Design review of the part built by this model. Coordinates are the model's own, in mm. A direction names the side the tool comes from. Coordinates: 2 decimals unless noted, no trailing zeros. Loops run counter-clockwise (first coordinate to the right, second up) from the corner with the lowest first, then second, coordinate; pieces in that order, holes last. Notation, with made-up numbers: (-7.5, -24) -> (41.5, -24) arc R26 cw to (41.5, 13) -> close; hole circle Ø10 at (2.5, 0.25). An arc over 180 degrees is marked (long way). Use a Markdown table: item, result. Add a question column.
Q1. Draft analysis for pull direction Z (two halves, no side actions). For faces 5 (the face through (-18.66, -201.37, -54.34)), 6 (the face through (-15.28, -209.38, -38.51)), 7 (the face through (-18.459, -209, -43)), state which applies: pulls with the +Z half, pulls with the -Z half, needs draft (parallel to the pull), parting line crosses it, or undercut.
Q2. Take a section at C-C on x = -14.5. Write out the cut boundary in (y, z).
Q3. Clearance check with flat-ended pins moving along their axes: pin 1 Ø3 at (x, z) = (-15, -40.5) entering from +Y; pin 2 Ø4 at (y, z) = (-213, -53.24) entering from +X; pin 3 Ø1.6 at (x, z) = (-17.5, -53) entering from -Y; pin 4 Ø3 at (y, z) = (-210.8, -39.24) entering from +X. State where each tip first meets the part, or that it passes through.
Q4. For faces 1 (the face through (-26.009, -211, -41)), 2 (the face through (-18.9, -210, -53.4)), 3 (the face through (-20.2, -203.8, -53.8)), 4 (the face through (-16.332, -203.496, -52.893)), list the 3-axis set-ups (+Z, -Z, +X, -X, +Y, -Y) from which the entire face can be reached by the end or side of a thin tool; tool diameter is ignored.
Q5. Take a section at D-D on z = -61.25. Write out the cut boundary in (x, y).
Q6. Take a section at A-A on y = -210.8. Write out the cut boundary in (x, z).
Q7. Take a section at B-B on z = -39. Write out the cut boundary in (x, y), plus the area to 3 significant figures.
Q8. For probe 1 along X at (y, z) = (-213.5, -39); probe 2 along Z at (x, y) = (-23.75, -210.8); probe 3 along Y at (x, z) = (-16.5, -58.25), list the stretches that pass through material, from the lowest coordinate up.
from build123d import *

# Parameters (mm, degrees)
MAIN_PROFILE_SKETCH_R          = 1.15
MAIN_EXTRUSION_DEPTH           = 3.6
DETAIL_PROFILE_2_SKETCH_R      = 2.7
DETAIL_EXTRUSION_2_DEPTH       = 0.6
DETAIL_PROFILE_3_SKETCH_R      = 1.15
DETAIL_EXTRUSION_3_DEPTH       = 2.2
DETAIL_EXTRUSION_4_DEPTH       = 1.2
DETAIL_EXTRUSION_5_DEPTH       = 2.8
DETAIL_EXTRUSION_6_DEPTH       = 4.4
ADAPTER_CROSS_BORE_1_PROFILE_R = 1.8
ADAPTER_CROSS_BORE_1_DEPTH     = 28
ADAPTER_CROSS_BORE_2_PROFILE_R = 1.6
ADAPTER_CROSS_BORE_2_DEPTH     = 16


with BuildPart() as part:
    # Main Profile Sketch → Main Extrusion (new body)
    with BuildSketch(Plane(origin=(0, -199.6, 0), x_dir=(-1, 0, 0), z_dir=(0, -1, 0))):
        with Locations(Location((19.009182883, 53.244882879, 0), (0, 0, 90))):
            Circle(MAIN_PROFILE_SKETCH_R)
    extrude(amount=MAIN_EXTRUSION_DEPTH)

    # Detail Profile 2 Sketch → Detail Extrusion 2 (add)
    with BuildSketch(Plane(origin=(0, -203.2, 0), x_dir=(-1, 0, 0), z_dir=(0, -1, 0))):
        with Locations(Location((19.009182883, 53.244882879, 0), (0, 0, 90))):
            Circle(DETAIL_PROFILE_2_SKETCH_R)
    extrude(amount=DETAIL_EXTRUSION_2_DEPTH)

    # Detail Profile 3 Sketch → Detail Extrusion 3 (add)
    with BuildSketch(Plane(origin=(0, -203.8, 0), x_dir=(-1, 0, 0), z_dir=(0, -1, 0))):
        with Locations(Location((19.009182883, 53.244882879, 0), (0, 0, 90))):
            Circle(DETAIL_PROFILE_3_SKETCH_R)
    extrude(amount=DETAIL_EXTRUSION_3_DEPTH)

    # Detail Profile 4 Sketch → Detail Extrusion 4 (add)
    with BuildSketch(Plane(origin=(0, -206, 0), x_dir=(-1, 0, 0), z_dir=(0, -1, 0))):
        with BuildLine():
            Line((18.459182883, 53.244882879), (18.459182883, 40.756988741))
            ThreePointArc((18.459182883, 40.756988741), (19.009182883, 65.744882879), (19.559182883, 40.756988741))
            Line((19.559182883, 40.756988741), (19.559182883, 53.244882879))
            Line((19.559182883, 53.244882879), (18.459182883, 53.244882879))
        make_face()
    extrude(amount=DETAIL_EXTRUSION_4_DEPTH)

    # Detail Profile 5 Sketch → Detail Extrusion 5 (add)
    with BuildSketch(Plane(origin=(0, -207.2, 0), x_dir=(-1, 0, 0), z_dir=(0, -1, 0))):
        with BuildLine():
            Line((12.009182883, 42.88872529), (12.009182883, 36.444882879))
            Line((12.009182883, 36.444882879), (18.459182883, 36.444882879))
            Line((18.459182883, 36.444882879), (18.459182883, 53.244882879))
            Line((18.459182883, 53.244882879), (19.559182883, 53.244882879))
            Line((19.559182883, 53.244882879), (19.559182883, 36.444882879))
            Line((19.559182883, 36.444882879), (26.009182883, 36.444882879))
            Line((26.009182883, 36.444882879), (26.009182883, 42.88872529))
            ThreePointArc((26.009182883, 42.88872529), (19.009182883, 65.744882879), (12.009182883, 42.88872529))
        make_face()
    extrude(amount=DETAIL_EXTRUSION_5_DEPTH)

    # Detail Profile 6 Sketch → Detail Extrusion 6 (add)
    with BuildSketch(Plane(origin=(0, -210, 0), x_dir=(-1, 0, 0), z_dir=(0, -1, 0))):
        with BuildLine():
            Line((12.009182883, 42.88872529), (12.009182883, 36.444882879))
            Line((12.009182883, 36.444882879), (18.459182883, 36.444882879))
            Line((18.459182883, 36.444882879), (18.459182883, 44.261704154))
            ThreePointArc((18.459182883, 44.261704154), (19.009182883, 62.244882879), (19.559182883, 44.261704154))
            Line((19.559182883, 44.261704154), (19.559182883, 36.444882879))
            Line((19.559182883, 36.444882879), (26.009182883, 36.444882879))
            Line((26.009182883, 36.444882879), (26.009182883, 42.88872529))
            ThreePointArc((26.009182883, 42.88872529), (19.009182883, 65.744882879), (12.009182883, 42.88872529))
        make_face()
    extrude(amount=DETAIL_EXTRUSION_6_DEPTH)

    # Adapter Cross Bore 1 profile → Adapter Cross Bore 1 (cut)
    with BuildSketch(Plane(origin=(-33.009182883, 0, 0), x_dir=(0, 0, -1), z_dir=(1, 0, 0))):
        with Locations((53.244882879, -213)):
            Circle(ADAPTER_CROSS_BORE_1_PROFILE_R)
    extrude(amount=ADAPTER_CROSS_BORE_1_DEPTH, mode=Mode.SUBTRACT)

    # Adapter Cross Bore 2 profile → Adapter Cross Bore 2 (cut)
    with BuildSketch(Plane(origin=(-27.009182883, 0, 0), x_dir=(0, 0, -1), z_dir=(1, 0, 0))):
        with Locations(Location((39.244882879, -210.8, 0), (0, 0, 180))):
            Circle(ADAPTER_CROSS_BORE_2_PROFILE_R)
    extrude(amount=ADAPTER_CROSS_BORE_2_DEPTH, mode=Mode.SUBTRACT)


solid = part.part
Answer list:
| question | item | result |
|---|---|---|
| 1 | face 5 | parting line crosses it |
| 1 | face 6 | undercut |
| 1 | face 7 | needs draft |
| 2 | outline | (-214.4, -64.9) -> (-206, -64.9) -> (-206, -41.59) -> (-207.2, -41.59) -> (-207.2, -36.44) -> (-214.4, -36.44) -> (-214.4, -45.46) -> (-210, -45.46) -> (-210, -61.03) -> (-214.4, -61.03) -> close; hole circle Ø3.2 at (-210.8, -39.24) |
| 3 | pin 1 | y = -206 |
| 3 | pin 2 | x = -6.51 |
| 3 | pin 3 | y = -210 |
| 3 | pin 4 | through |
| 4 | face 1 | +Z, -X, +Y, -Y |
| 4 | face 2 | -Y |
| 4 | face 3 | none |
| 4 | face 4 | +Y |
| 5 | outline | (-28.61, -214.4) -> (-23.12, -214.4) -> (-23.12, -210) -> (-14.9, -210) -> (-14.9, -214.4) -> (-9.41, -214.4) -> (-9.41, -206) -> (-28.61, -206) -> close |
| 6 | outline | (-26.01, -42.89) arc R12.5 ccw (long way) to (-12.01, -42.89) -> (-12.01, -40.84) -> (-18.46, -40.84) -> (-18.46, -44.26) arc R9 cw (long way) to (-19.56, -44.26) -> (-19.56, -40.84) -> (-26.01, -40.84) -> close; (-26.01, -37.64) -> (-19.56, -37.64) -> (-19.56, -36.44) -> (-26.01, -36.44) -> close; (-18.46, -37.64) -> (-12.01, -37.64) -> (-12.01, -36.44) -> (-18.46, -36.44) -> close |
| 7 | outline | (-26.01, -214.4) -> (-19.56, -214.4) -> (-19.56, -212.38) -> (-26.01, -212.38) -> close; (-26.01, -209.22) -> (-19.56, -209.22) -> (-19.56, -207.2) -> (-26.01, -207.2) -> close; (-18.46, -214.4) -> (-12.01, -214.4) -> (-12.01, -212.38) -> (-18.46, -212.38) -> close; (-18.46, -209.22) -> (-12.01, -209.22) -> (-12.01, -207.2) -> (-18.46, -207.2) -> close |
| 7 | area | 52.1 mm² |
| 8 | probe 1 | -26.01 to -19.56, -18.46 to -12.01 |
| 8 | probe 2 | -64.81 to -60.9, -45.59 to -40.84, -37.64 to -36.44 |
| 8 | probe 3 | -210 to -206 |
